from build123d import *

# Parameters (mm, degrees)
BOSS_EXTRU_1_DEPTH      = 0.4
BOSS_EXTRU_1_DEPTH_BACK = 10.6
ESQUISSE1_R             = 8
ESQUISSE1_R_2           = 2.5
ESQUISSE2_R             = 6.8
ESQUISSE2_R_2           = 4.3
ENL_V_MAT_EXTRU_1_DEPTH = 0.3


with BuildPart() as part:
    # Sketch1 → Revolve1 (revolve)
    with BuildSketch(Plane.XY, mode=Mode.PRIVATE) as revolve1_sk:
        Polygon((0.5, 7), (-0.5, 7), (-0.5, 8), (-5.1, 8), (-5.1, 9.8), (-2.95, 11.95), (2.95, 11.95), (5.1, 9.8), (5.1, 8), (0.5, 8), align=None)
    revolve(revolve1_sk.sketch.rotate(Axis((0, 0, 0), (-1, 0, 0)), 90), axis=Axis((0, 0, 0), (-1, 0, 0)))

    # Esquisse1 → Boss.-Extru.1 (add, two sides: drawn at the far end of the back side and taken through both)
    with BuildSketch(Plane.ZY.offset(5.1).offset(-BOSS_EXTRU_1_DEPTH_BACK)):
        Circle(ESQUISSE1_R)
        Circle(ESQUISSE1_R_2, mode=Mode.SUBTRACT)
    extrude(amount=BOSS_EXTRU_1_DEPTH + BOSS_EXTRU_1_DEPTH_BACK)

    # Esquisse2 → Enlèv. mat.-Extru.1 (cut)
    with BuildSketch(Plane.ZY.offset(5.5)):
        Circle(ESQUISSE2_R)
        Circle(ESQUISSE2_R_2, mode=Mode.SUBTRACT)
    enl_v_mat_extru_1 = extrude(amount=-ENL_V_MAT_EXTRU_1_DEPTH, mode=Mode.SUBTRACT)

    # Symétrie1: Enlèv. mat.-Extru.1 across plane
    add(enl_v_mat_extru_1.mirror(Plane(origin=(0, 0, 0), x_dir=(0, 0, 1), z_dir=(1, 0, 0))), mode=Mode.SUBTRACT)


solid = part.part
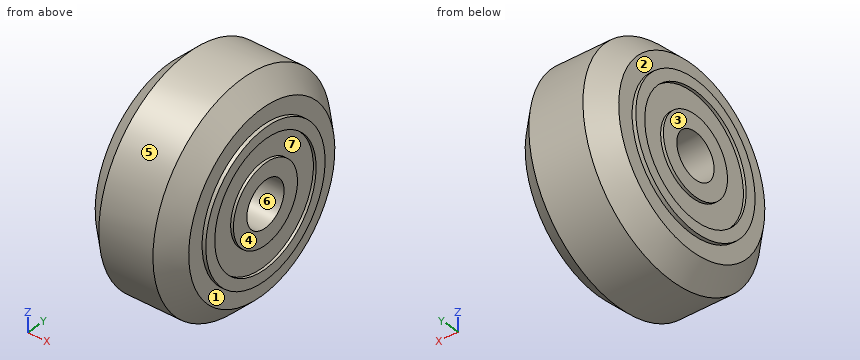
Could you check a few things on this model? Use its own coordinates, in mm. Face numbers are marked on the shaded views. A direction names the side the tool comes from. Coordinates: 2 decimals unless noted, no trailing zeros. Loops run counter-clockwise (first coordinate to the right, second up) from the corner with the lowest first, then second, coordinate; pieces in that order, holes last.
1. I need wall thicknesses on L1, parallel to Y at x = 5.35, z = 0; L2, parallel to Y at x = 0, z = 0; L3, parallel to X at y = 3.75, z = -2.75. Which ranges of each line are inside material? Lowest first, please.
2. We'd pull the mould along Z, two halves only. Please class the marked faces 4, 5, 6 and 7: released by +Z, released by -Z, zero draft, split by the parting line, or undercut.
3. For P1, Ø4, axis at x = 0.5, y = 7.5, coming from the -Z side; P2, Ø4, axis at x = 1, y = 5, coming from the +Z side; P3, Ø4, axis at x = 4.5, y = 5, coming from the +Z side, each with a flat end and sliding along its axis, tell me the tip position at first contact or that it passes through.
4. Imagine slicing it at A-A (x = -3.25). Please give me the cut outline in (y, z), and give its area (3 significant figures).
5. Imagine slicing it at B-B (x = 1.25). Please give me the cut outline in (y, z), and give its area (3 significant figures).
6. For the marked faces 1, 2 and 3, which set-ups out of +Z, -Z, +X, -X, +Y, -Y let a thin tool reach every point of the face, with its end or its side?
Computed values:
1. L1: y = -8 to -6.8, -4.3 to -2.5, 2.5 to 4.3, 6.8 to 8
1. L2: y = -11.95 to -2.5, 2.5 to 11.95
1. L3: x = -5.2 to 5.2
2. face 4: zero draft
2. face 5: split by the parting line
2. face 6: undercut
2. face 7: undercut
3. P1: stops at z = -10.61
3. P2: stops at z = 11.57
3. P3: stops at z = 11.35
4. outline: circle Ø23.3 at (0, 0); hole circle Ø5 at (0, 0)
4. area: 407 mm2
5. outline: circle Ø23.9 at (0, 0); hole circle Ø5 at (0, 0)
5. area: 429 mm2
6. face 1: +X
6. face 2: -X
6. face 3: +Z, -Z, -X, +Y, -Y
